from build123d import *

# Parameters (mm, degrees)
SKETCH1_W           = 145
SKETCH1_H           = 65
BOSS_EXTRUDE1_DEPTH = 11
SKETCH2_W           = 50
SKETCH2_H           = 65
CUT_EXTRUDE1_DEPTH  = 20.5


with BuildPart() as part:
    # Sketch1 → Boss-Extrude1 (new body, symmetric)
    with BuildSketch(Plane(origin=(0, 0, 0), x_dir=(1, 0, 0), z_dir=(0, 1, 0))):
        Rectangle(SKETCH1_W, SKETCH1_H)
    extrude(amount=BOSS_EXTRUDE1_DEPTH, both=True)

    # Sketch2 → Cut-Extrude1 (cut)
    with BuildSketch(Plane(origin=(0, 11, 0), x_dir=(1, 0, 0), z_dir=(0, 1, 0))):
        with Locations((-27.5, 0)):
            Rectangle(SKETCH2_W, SKETCH2_H)
    extrude(amount=-CUT_EXTRUDE1_DEPTH, mode=Mode.SUBTRACT)


solid = part.part
Check sheet for the modelled part. Datum: model origin and axes. Units: mm. A direction names the side the tool comes from. Round coordinates to 2 decimals unless told otherwise and drop trailing zeros. Order: outer loops, then holes, each group sorted by start corner. A loop starts at its lowest first (then second) coordinate and runs counter-clockwise, first axis right, second up.
(1) Access from +Z, -Z, +X, -X, +Y, -Y to the whole of each face (thin tool, end or side, straight path). Record for faces 4 (the flat face through (-52.5, 1, 0)), 5 (the flat face through (72.5, 0, 0)).
(2) Scan lines: probe 1 along X at (y, z) = (-5, -3.5); probe 2 along Y at (x, z) = (-41, 19). Record each from-to range of solid material in increasing order.
(3) Cross-section at A-A, the plane y = 0.5. Enter the section's corners in (x, z), and give its area (4 significant figures).
(4) Draft check along X on faces 1 (the flat face through (-1, -11, 0)), 2 (the flat face through (-2.5, 1, 0)), 3 (the flat face through (-72.5, 0, 0)). Enter one of: pulls with the +X half, pulls with the -X half, needs draft (parallel to the pull), parting line crosses it, or undercut.
(5) Cross-section at B-B, the plane z = -7.5. Enter the section's corners in (x, y), and give its area (4 significant figures).
(6) Cross-section at C-C, the plane x = -49.5. Enter the section's corners in (y, z), and give its area (3 significant figures).
Check sheet entries:
1. face 4: +Z, -Z, +Y
1. face 5: +Z, -Z, +X, +Y, -Y
2. probe 1: x = -72.5 to -52.5, -2.5 to 72.5
2. probe 2: y = -11 to -9.5
3. outline: (-72.5, -32.5) - (-52.5, -32.5) - (-52.5, 32.5) - (-72.5, 32.5) - close; (-2.5, -32.5) - (72.5, -32.5) - (72.5, 32.5) - (-2.5, 32.5) - close
3. area: 6,175 mm2
4. face 1: needs draft
4. face 2: undercut
4. face 3: pulls with the -X half
5. outline: (-72.5, -11) - (72.5, -11) - (72.5, 11) - (-2.5, 11) - (-2.5, -9.5) - (-52.5, -9.5) - (-52.5, 11) - (-72.5, 11) - close
5. area: 2,165 mm2
6. outline: (-11, -32.5) - (-9.5, -32.5) - (-9.5, 32.5) - (-11, 32.5) - close
6. area: 97.5 mm2
